from build123d import *

# Parameters (mm, degrees)
F0_R          = 2.5
F1_DEPTH      = 6
F3_R          = 2.15
F1_FACE_R     = 2.5
F6_R          = 3
F7_DEPTH      = 1
F9_R          = 0.75
F10_DEPTH     = 8.0010001
F12_W         = 3
F12_H         = 0.3
F13_DEPTH     = 3
F14_T4_DEPTH  = 4.4618227718
F14_S5_R      = 2.5
F14_T6_DEPTH  = 4
F14_S7_R      = 0.75
F14_T8_DEPTH  = 4
F14_T12_DEPTH = 4.1272739781
F14_S13_R     = 2.5
F14_T14_DEPTH = 4
F14_S15_R     = 0.75
F14_T16_DEPTH = 4
F14_T20_DEPTH = 4.4618227718
F14_S21_R     = 2.5
F14_T22_DEPTH = 4
F14_S23_R     = 0.75
F14_T24_DEPTH = 4
F14_T28_DEPTH = 4.1272739781
F14_S29_R     = 2.5
F14_T30_DEPTH = 4
F14_S31_R     = 0.75
F14_T32_DEPTH = 4


# Not quite as in the source:
# - a fillet or chamfer that OpenCascade refuses, or shapes differently, is made with other operations: its cross-section is extruded or revolved along the edge and cut away or added


with BuildPart() as f1:
    # F0 (on Front) → F1 (new body)
    with BuildSketch(Plane.XZ):
        Circle(F0_R)
    extrude(amount=F1_DEPTH)

    # F3 (on offset) → F4 section 0
    with BuildSketch(Plane.XZ.offset(7)):
        Circle(F3_R)
    # F1_face (on face) → F4 section 1
    with BuildSketch(Plane.XZ.offset(6)):
        Circle(F1_FACE_R)
    loft()

    # F6 (on offset) → F7 (join)
    with BuildSketch(Plane(origin=(0, 0, 0), x_dir=(-1, 0, 0), z_dir=(0, 1, 0))):
        Circle(F6_R)
    extrude(amount=F7_DEPTH)

    # F9 (on offset) → F10 (cut, through all)
    with BuildSketch(Plane(origin=(0, 1, 0), x_dir=(-1, 0, 0), z_dir=(0, 1, 0))):
        with Locations((0.1672743968, 0)):
            Circle(F9_R)
    extrude(amount=-F10_DEPTH, mode=Mode.SUBTRACT)

    # F12 (on offset) → F13 (cut)
    with BuildSketch(Plane.XZ.offset(7)):
        with Locations((1.5, 0.15)):
            Rectangle(F12_W, F12_H)
        Polygon((3, 0), (0, 0), (0, 0.3), (-3, 0.3), (-3, 0), (-3, -0.3), (0, -0.3), (3, -0.3), align=None)
    extrude(amount=-F13_DEPTH, mode=Mode.SUBTRACT)

    # F14: fillet of radius 0.5 on 4 edges, made by hand


with BuildPart() as f14_tool2:
    # F14_s3 → F14_t4 (new body)
    with BuildSketch(Plane.YZ.offset(-0.7298880426)):
        with BuildLine():
            ThreePointArc((-4, 0.2), (-4.1464466094, -0.1535533906), (-4.5, -0.3))
            Line((-4.5, -0.3), (-4, -0.3))
            Line((-4, -0.3), (-4, 0.2))
        make_face()
    extrude(amount=F14_T4_DEPTH)

    # F14_s5 → F14_t6 (intersect, symmetric)
    with BuildSketch(Plane.XZ.offset(4.2)):
        Circle(F14_S5_R)
    extrude(amount=F14_T6_DEPTH, both=True, mode=Mode.INTERSECT)

    # F14_s7 → F14_t8 (cut, symmetric)
    with BuildSketch(Plane.XZ.offset(4.2)):
        with Locations((-0.1672743968, 0)):
            Circle(F14_S7_R)
    extrude(amount=F14_T8_DEPTH, both=True, mode=Mode.SUBTRACT)


with BuildPart() as f1_1:
    add(f1.part)

    # F14_t1: union F14_tool2
    add(f14_tool2.part)


with BuildPart() as f14_tool10:
    # F14_s11 → F14_t12 (new body)
    with BuildSketch(Plane.YZ.offset(-3.7319347292)):
        with BuildLine():
            ThreePointArc((-4.5, -0.3), (-4.1464466094, -0.1535533906), (-4, 0.2))
            Line((-4, 0.2), (-4, -0.3))
            Line((-4, -0.3), (-4.5, -0.3))
        make_face()
    extrude(amount=F14_T12_DEPTH)

    # F14_s13 → F14_t14 (intersect, symmetric)
    with BuildSketch(Plane.XZ.offset(4.2)):
        Circle(F14_S13_R)
    extrude(amount=F14_T14_DEPTH, both=True, mode=Mode.INTERSECT)

    # F14_s15 → F14_t16 (cut, symmetric)
    with BuildSketch(Plane.XZ.offset(4.2)):
        with Locations((-0.1672743968, 0)):
            Circle(F14_S15_R)
    extrude(amount=F14_T16_DEPTH, both=True, mode=Mode.SUBTRACT)


with BuildPart() as f1_2:
    add(f1_1.part)

    # F14_t9: union F14_tool10
    add(f14_tool10.part)


with BuildPart() as f14_tool18:
    # F14_s19 → F14_t20 (new body)
    with BuildSketch(Plane.YZ.offset(3.7319347292)):
        with BuildLine():
            ThreePointArc((-4, -0.2), (-4.1464466094, 0.1535533906), (-4.5, 0.3))
            Line((-4.5, 0.3), (-4, 0.3))
            Line((-4, 0.3), (-4, -0.2))
        make_face()
    extrude(amount=-F14_T20_DEPTH)

    # F14_s21 → F14_t22 (intersect, symmetric)
    with BuildSketch(Plane.XZ.offset(4.2)):
        Circle(F14_S21_R)
    extrude(amount=F14_T22_DEPTH, both=True, mode=Mode.INTERSECT)

    # F14_s23 → F14_t24 (cut, symmetric)
    with BuildSketch(Plane.XZ.offset(4.2)):
        with Locations((-0.1672743968, 0)):
            Circle(F14_S23_R)
    extrude(amount=F14_T24_DEPTH, both=True, mode=Mode.SUBTRACT)


with BuildPart() as f1_3:
    add(f1_2.part)

    # F14_t17: union F14_tool18
    add(f14_tool18.part)


with BuildPart() as f14_tool26:
    # F14_s27 → F14_t28 (new body)
    with BuildSketch(Plane.YZ.offset(0.3953392489)):
        with BuildLine():
            ThreePointArc((-4, -0.2), (-4.1464466094, 0.1535533906), (-4.5, 0.3))
            Line((-4.5, 0.3), (-4, 0.3))
            Line((-4, 0.3), (-4, -0.2))
        make_face()
    extrude(amount=-F14_T28_DEPTH)

    # F14_s29 → F14_t30 (intersect, symmetric)
    with BuildSketch(Plane.XZ.offset(4.2)):
        Circle(F14_S29_R)
    extrude(amount=F14_T30_DEPTH, both=True, mode=Mode.INTERSECT)

    # F14_s31 → F14_t32 (cut, symmetric)
    with BuildSketch(Plane.XZ.offset(4.2)):
        with Locations((-0.1672743968, 0)):
            Circle(F14_S31_R)
    extrude(amount=F14_T32_DEPTH, both=True, mode=Mode.SUBTRACT)


with BuildPart() as f1_4:
    add(f1_3.part)

    # F14_t25: union F14_tool26
    add(f14_tool26.part)


solid = f1_4.part
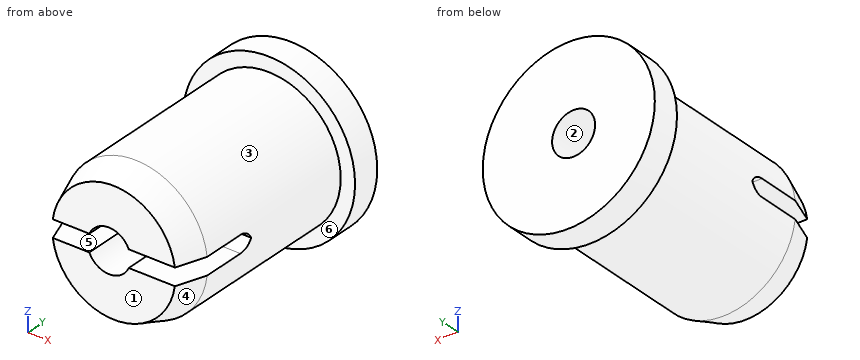
The listing builds one solid part. Answer for the finished solid, in the listing's coordinates (mm). Face numbers are marked on the shaded views. A direction names the side the tool comes from. Give positions to 0.01 mm unless a question says otherwise; leave off trailing zeros. Order: outer loops, then holes, each group sorted by start corner. A loop starts at its lowest first (then second) coordinate and runs counter-clockwise, first axis right, second up. Notation, with made-up numbers: (65, 22) - (122, 22) arc R14 ccw to (122, 32) - close; hole circle Ø3 at (57.5, -37.5). An arc over 180 degrees is marked (long way). Use one line per item in the form item = value.
1) The mould has two halves that part along Z. Classify the marked faces 1, 2 and 3: released by +Z, released by -Z, zero draft, split by the parting line, or undercut.
Verdict:
face_1 = zero draft
face_2 = undercut
face_3 = split by the parting line
2) Find section A-A on x = 0. Determine the outline of the cut face in (y, z).
Verdict:
outline = (-7, -2.15) - (-6, -2.5) - (0, -2.5) - (0, -3) - (1, -3) - (1, -0.73) - (-7, -0.73) - close; (-7, 0.73) - (1, 0.73) - (1, 3) - (0, 3) - (0, 2.5) - (-6, 2.5) - (-7, 2.15) - close
3) Find section B-B on y = -0.5. Determine the outline of the cut face in (x, z), and give its area (3 significant figures).
Verdict:
outline = circle Ø5 at (0, 0); hole circle Ø1.5 at (-0.17, 0)
area = 17.9 mm^2
4) Each of these flat-tipped pins is pushed along its axis until it touches: pin 1 (0.6 mm diameter, centred on x = 2, y = -6, fed in from -Z); pin 2 (2 mm diameter, centred on x = -0.17, z = 0, fed in from -Y); pin 3 (1.3 mm diameter, centred on x = -1.5, y = -6, fed in from +Z); pin 4 (1 mm diameter, centred on x = 2, y = -2, fed in from -Z). Where does it stop, or does it pass through?
Verdict:
pin_1 = -1.83
pin_2 = -7
pin_3 = 2.35
pin_4 = -2
5) Consider probe 1 along Y at (x, z) = (1.95, -1.7); probe 2 along Z at (x, y) = (0.3, 0.25); probe 3 along Z at (x, y) = (2.1, -6.5). Determine where each line is inside the solid, lowest interval first. Write a range as [from, to].
Verdict:
probe_1 = [0, 1]
probe_2 = [-2.98, -0.59], [0.59, 2.98]
probe_3 = [-1, -0.3], [0.3, 1]
6) For the marked faces 4, 5 and 6, determine the directions among +Z, -Z, +X, -X, +Y, -Y from which every point of the face is accessible in a straight line to the end or side of a thin tool.
Verdict:
face_4 = -Z, -Y
face_5 = +X, -X, -Y
face_6 = -Y
